from build123d import *

# Parameters (mm, degrees)
SKETCH_2_W          = 76
SKETCH_2_H          = 41
EXTRUDE_1_DEPTH     = 50
CUT_EXTRUDE_1_REACH = 102
SKETCH_3_R          = 2.2


with BuildPart() as part:
    # 草图2 → 凸台-拉伸1 (new body)
    with BuildSketch(Plane(origin=(0, 0, 0), x_dir=(1, 0, 0), z_dir=(0, 1, 0))):
        Polygon((-38, -26.5), (44, -26.5), (44, 26.5), (-38, 26.5), (-56, 26.5), (-56, -26.5), align=None)
        Rectangle(SKETCH_2_W, SKETCH_2_H, mode=Mode.SUBTRACT)
    extrude(amount=EXTRUDE_1_DEPTH)

    # 草图3 → 切除-拉伸1 (cut, up to next)
    with BuildSketch(Plane(origin=(44, 0, 0), x_dir=(0, 0, -1), z_dir=(1, 0, 0)), mode=Mode.PRIVATE) as cut_extrude_1_sk1:
        with Locations((0, 25)):
            Circle(SKETCH_3_R)
    cut_extrude_1_tool1 = extrude(cut_extrude_1_sk1.sketch, amount=-CUT_EXTRUDE_1_REACH, mode=Mode.PRIVATE) & part.part
    add(cut_extrude_1_tool1.solids().sort_by_distance((44, 25, 0))[0], mode=Mode.SUBTRACT)


solid = part.part
Input: part model. Units: mm. Frame: model coordinates. A direction names the side the tool comes from. Coordinates: 2 decimals unless noted, no trailing zeros. Order: outer loops, then holes, each group sorted by start corner. A loop starts at its lowest first (then second) coordinate and runs counter-clockwise, first axis right, second up. Notation, with made-up numbers: M 61,2 L 113,2 A7 ccw 113,8 Z; hole C 25.25,4.25 d9. An arc over 180 degrees is marked long. Answer in a Markdown table with one row per item.
(1) Section query B-B, the plane z = 0. Output: boundary loops of the cut face in (x, y), plus the area to 3 significant figures.
Numbers:
| item | result |
|---|---|
| outline | M -56,0 L -38,0 L -38,50 L -56,50 Z; M 38,0 L 44,0 L 44,22.8 L 38,22.8 Z; M 38,27.2 L 44,27.2 L 44,50 L 38,50 Z |
| area | 1,170 mm^2 |
(2) Section query C-C, the plane y = 25. Output: boundary loops of the cut face in (x, z), plus the area to 3 significant figures.
Numbers:
| item | result |
|---|---|
| outline | M -56,-26.5 L 44,-26.5 L 44,-2.2 L 38,-2.2 L 38,-20.5 L -38,-20.5 L -38,20.5 L 38,20.5 L 38,2.2 L 44,2.2 L 44,26.5 L -56,26.5 Z |
| area | 2,160 mm^2 |
(3) Section query A-A, the plane x = 34.5. Output: boundary loops of the cut face in (y, z), plus the area to 3 significant figures.
Numbers:
| item | result |
|---|---|
| outline | M 0,-26.5 L 50,-26.5 L 50,-20.5 L 0,-20.5 Z; M 0,20.5 L 50,20.5 L 50,26.5 L 0,26.5 Z |
| area | 600 mm^2 |
(4) Access query for faces 5 (the flat face through (-1, 25, -20.5)), 6 (the flat face through (-40, 0, 0)). Directions: +Z, -Z, +X, -X, +Y, -Y. A direction counts if a zero-diameter tool reaches every point of the face in a straight line with its end or side. Return the directions, or none.
Numbers:
| item | result |
|---|---|
| face 5 | +Y, -Y |
| face 6 | +Z, -Z, +X, -X, -Y |
(5) Material intervals for line 1 (Y direction, x = 41, z = 0); line 2 (X direction, y = 37, z = 17); line 3 (Z direction, x = -6, y = 3), sorted ascending. Write a range as [from, to].
Numbers:
| item | result |
|---|---|
| line 1 | y = [0, 22.8], [27.2, 50] |
| line 2 | x = [-56, -38], [38, 44] |
| line 3 | z = [-26.5, -20.5], [20.5, 26.5] |
(6) Draft query along X for faces 1 (the flat face through (44, 19, 0)), 2 (the flat face through (-56, 25, 0)), 3 (the flat face through (-38, 25, 0)), 4 (the cylindrical face through (41.042, 22.852, 0.477)). Return one class per face: pulls with the +X half, pulls with the -X half, needs draft (parallel to the pull), parting line crosses it, or undercut.
Numbers:
| item | result |
|---|---|
| face 1 | pulls with the +X half |
| face 2 | pulls with the -X half |
| face 3 | undercut |
| face 4 | needs draft |
(7) Section query D-D, the plane z = 12. Output: boundary loops of the cut face in (x, y).
Numbers:
| item | result |
|---|---|
| outline | M -56,0 L -38,0 L -38,50 L -56,50 Z; M 38,0 L 44,0 L 44,50 L 38,50 Z |
